Verification items for the finished model (mm, model axes). Face numbers are marked on the shaded views. A direction names the side the tool comes from. Coordinates: 2 decimals unless noted, no trailing zeros. Write each loop counter-clockwise with the first axis right and the second up, starting at its lowest first coordinate (ties: lowest second). Pieces come first, ordered by that corner, then holes.
```python
from build123d import *

# Parameters (mm, degrees)
SKETCH3_R           = 2.38125
BOSS_EXTRUDE1_DEPTH = 3.556
CUT_EXTRUDE1_START  = -3.4798
SKETCH4_R           = 2.38125
CUT_EXTRUDE1_DEPTH  = 3.4798


with BuildPart() as part:
    # Sketch3 → Boss-Extrude1 (new body)
    with BuildSketch(Plane(origin=(0, 0, 0), x_dir=(1, 0, 0), z_dir=(0, 1, 0))):
        with BuildLine():
            Line((5.654009559, -2.890445624), (8.020116475, -2.890445624))
            Line((8.020116475, -2.890445624), (10.386223391, -2.890445624))
            Line((10.386223391, -2.890445624), (10.386223391, 2.890445624))
            Line((10.386223391, 2.890445624), (8.020116475, 2.890445624))
            Line((8.020116475, 2.890445624), (5.654009559, 2.890445624))
            ThreePointArc((5.654009559, 2.890445624), (-6.35, 0), (5.654009559, -2.890445624))
        make_face()
        with Locations(Location((0, 0, 0), (0, 0, 270))):
            Circle(SKETCH3_R, mode=Mode.SUBTRACT)
    extrude(amount=-BOSS_EXTRUDE1_DEPTH)

    # Sketch4 → Cut-Extrude1 (cut)
    with BuildSketch(Plane(origin=(0, -3.556, 0), x_dir=(-1, 0, 0), z_dir=(0, -1, 0)).offset(CUT_EXTRUDE1_START)):
        with BuildLine():
            ThreePointArc((4.936299023, -0.4064), (0.463581133, 4.931257602), (-4.925553828, 0.5207))
            Line((-4.925553828, 0.5207), (-7.402053828, 0.5207))
            Line((-7.402053828, 0.5207), (-9.878553828, 0.5207))
            Line((-9.878553828, 0.5207), (-9.878553828, -0.5207))
            Line((-9.878553828, -0.5207), (-7.402053828, -0.5207))
            Line((-7.402053828, -0.5207), (-4.925553828, -0.5207))
            ThreePointArc((-4.925553828, -0.5207), (0.05740198, -4.952667363), (4.936299023, -0.4064))
        make_face()
        with Locations(Location((0, 0, 0), (0, 0, 270))):
            Circle(SKETCH4_R, mode=Mode.SUBTRACT)
    extrude(amount=CUT_EXTRUDE1_DEPTH, mode=Mode.SUBTRACT)


solid = part.part
```
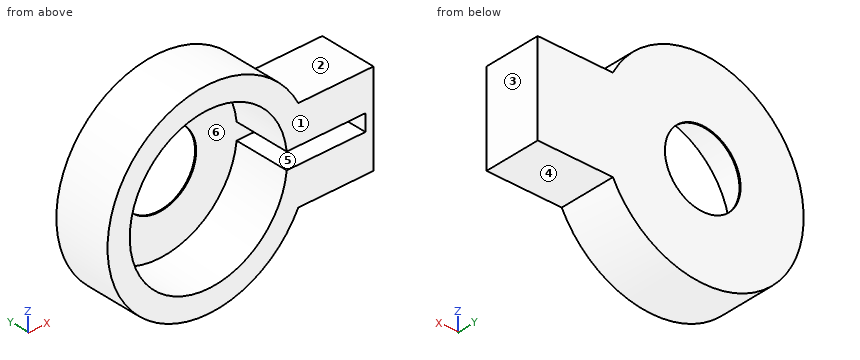
1. Sectioned sample at D-D, the plane x = 8. Record the boundary of the cut face in (y, z), and give its area (3 significant figures).
2. Draft check along X on the marked faces 3, 4, 5 and 6. Enter one of: pulls with the +X half, pulls with the -X half, needs draft (parallel to the pull), parting line crosses it, or undercut.
3. Gauge pin test, flat ends, axial feed: P1, Ø1.7, axis at x = 8.5, y = -2.5, coming from the -Z side; P2, Ø1, axis at y = -2, z = 3.5, coming from the -X side; P3, Ø1, axis at x = 6.5, y = -1.5, coming from the +Z side. Record the tip position at first contact, or that the pin passes through.
4. Tool access check on the marked faces 1 and 2. Record the directions out of +Z, -Z, +X, -X, +Y, -Y that give a thin tool (end or side, any length) a straight path to the whole face; none if there is none.
5. Sectioned sample at A-A, the plane y = -0.85. Record the boundary of the cut face in (x, z).
6. Sectioned sample at B-B, the plane x = 0. Record the boundary of the cut face in (y, z).
7. Sectioned sample at C-C, the plane z = 0. Record the boundary of the cut face in (x, y).
8. Material ranges on L1, parallel to Z at x = 8.75, y = -0.45; L2, parallel to X at y = -1.4, z = 2.5; L3, parallel to Z at x = -3.75, y = -2.85, recorded low to high.
Outcome:
1. outline: (-3.56, -2.89) - (0, -2.89) - (0, 2.89) - (-3.56, 2.89) - (-3.56, 0.52) - (-0.08, 0.52) - (-0.08, -0.52) - (-3.56, -0.52) - close
1. area: 16.9 mm2
2. face 3: pulls with the +X half
2. face 4: needs draft
2. face 5: undercut
2. face 6: undercut
3. P1: stops at z = -2.89
3. P2: stops at x = -5.6
3. P3: stops at z = 2.89
4. face 1: +Z, -Z, +X, -X, -Y
4. face 2: +Z, +X, +Y, -Y
5. outline: (5.65, -2.89) - (10.39, -2.89) - (10.39, 2.89) - (5.65, 2.89) arc R6.35 ccw (long way) to start; hole (4.93, -0.52) - (9.88, -0.52) - (9.88, 0.52) - (4.93, 0.52) arc R4.95 ccw (long way) to start
6. outline: (-3.56, -6.35) - (0, -6.35) - (0, -2.38) - (-0.08, -2.38) - (-0.08, -4.95) - (-3.56, -4.95) - close; (-3.56, 4.95) - (-0.08, 4.95) - (-0.08, 2.38) - (0, 2.38) - (0, 6.35) - (-3.56, 6.35) - close
7. outline: (-6.35, -3.56) - (-4.95, -3.56) - (-4.95, -0.08) - (-2.38, -0.08) - (-2.38, 0) - (-6.35, 0) - close; (2.38, -0.08) - (9.88, -0.08) - (9.88, -3.56) - (10.39, -3.56) - (10.39, 0) - (2.38, 0) - close
8. L1: z = -2.89 to -0.52, 0.52 to 2.89
8. L2: x = -5.84 to -4.28, 4.28 to 10.39
8. L3: z = -5.12 to -3.24, 3.24 to 5.12
